```python
from build123d import *

# Parameters (mm, degrees)
SKETCH_1_R      = 5
SKETCH_1_R_2    = 3
EXTRUDE_1_DEPTH = 4
EXTRUDE_START   = 4
SKETCH_1_3_R    = 5
SKETCH_1_3_R_2  = 3
EXTRUDE_2_DEPTH = 2


with BuildPart() as part:
    # 草图1 → 凸台-拉伸1 (new body)
    # profile 1 of 2: a face of its own
    with BuildSketch(Plane(origin=(0, 0, 0), x_dir=(1, 0, 0), z_dir=(0, 1, 0))):
        with Locations(Location((0, 0, 0), (0, 0, 270))):
            Circle(SKETCH_1_R)
        with Locations(Location((0, 0, 0), (0, 0, 270))):
            Circle(SKETCH_1_R_2, mode=Mode.SUBTRACT)
    # profile 2 of 2: a face of its own
    with BuildSketch(Plane(origin=(0, 0, 0), x_dir=(1, 0, 0), z_dir=(0, 1, 0))):
        with Locations(Location((0, 0, 0), (0, 0, 270))):
            Circle(SKETCH_1_R_2)
        with BuildLine():
            ThreePointArc((-2, 1.5), (0, -2.5), (2, 1.5))
            Line((2, 1.5), (-2, 1.5))
        make_face(mode=Mode.SUBTRACT)
    extrude(amount=EXTRUDE_1_DEPTH)

    # 草图1<3> → 凸台-拉伸2 (add)
    with BuildSketch(Plane(origin=(0, 0, 0), x_dir=(1, 0, 0), z_dir=(0, 1, 0)).offset(EXTRUDE_START)):
        with Locations(Location((0, 0, 0), (0, 0, 270))):
            Circle(SKETCH_1_3_R)
        with Locations(Location((0, 0, 0), (0, 0, 270))):
            Circle(SKETCH_1_3_R_2, mode=Mode.SUBTRACT)
    extrude(amount=EXTRUDE_2_DEPTH)


solid = part.part
```
Source: CAD feature listing. Evaluate the final solid. Frame: model axes, mm. A direction names the side the tool comes from. Give positions to 0.01 mm unless a question says otherwise; leave off trailing zeros. Write each loop counter-clockwise with the first axis right and the second up, starting at its lowest first coordinate (ties: lowest second). Pieces come first, ordered by that corner, then holes. Notation, with made-up numbers: (29.5, 36.25) - (61.5, 36.25) arc R7 ccw to (61.5, 40.25) - close; hole circle Ø2 at (-15.75, 7.5). An arc over 180 degrees is marked (long way). One line per item, written item: value. Start each with the question number.
Q1. Draft query along X for faces 1 (the face through (-0.1, 2, 2.5)), 2 (the face through (-4.88, 2.96, -1.08)), 3 (the face through (0, 0, -2)). Return one class per face: +X half, -X half, draft (parallel to the pull), parting line (faces both ways), or undercut.
Q2. Section query C-C, the plane y = 2.25. Return the cut outline in (x, z).
Q3. Section query D-D, the plane z = -2. Return the cut outline in (x, y).
Q4. Section query B-B, the plane x = -1.25. Return the cut outline in (y, z), then the cut area to 3 significant figures.
Q5. Section query A-A, the plane z = 0. Return the cut outline in (x, y), then the cut area to 3 significant figures.
Q6. Material intervals for probe 1 along X at (y, z) = (2.9, 0); probe 2 along X at (y, z) = (4.4, 0); probe 3 along Z at (x, y) = (0.25, 0.5), sorted ascending. Write a range as from..to.
Q7. Set-up query: faces 4 (the face through (0.9, 4.99, 2.86)), 5 (the face through (0, 2, -1.5)), 6 (the face through (-3.3, 6, -0.1)). Return all of +Z, -Z, +X, -X, +Y, -Y with unobstructed straight access to the full face (end or side cutting, diameter ignored); none if empty.
Q8. First-contact query: pin 1 Ø3 at (x, y) = (-2.5, 0.5) entering from +Z; pin 2 Ø3 at (y, z) = (2.5, -0.5) entering from -X; pin 3 Ø1 at (y, z) = (4.5, -2) entering from -X. Flat tips, straight axial feed; report the tip coordinate or a pass-through.
Answer:
1. face 1: undercut
1. face 2: parting line
1. face 3: draft
2. outline: circle Ø10 at (0, 0); hole (-2, -1.5) - (2, -1.5) arc R2.5 ccw (long way) to start
3. outline: (-4.58, 0) - (4.58, 0) - (4.58, 6) - (2.24, 6) - (2.24, 4) - (-2.24, 4) - (-2.24, 6) - (-4.58, 6) - close
4. outline: (0, -4.84) - (6, -4.84) - (6, -2.73) - (4, -2.73) - (4, -1.5) - (0, -1.5) - close; (0, 2.17) - (4, 2.17) - (4, 2.73) - (6, 2.73) - (6, 4.84) - (0, 4.84) - close
4. area: 32.5 mm2
5. outline: (-5, 0) - (-2.5, 0) - (-2.5, 4) - (-3, 4) - (-3, 6) - (-5, 6) - close; (2.5, 0) - (5, 0) - (5, 6) - (3, 6) - (3, 4) - (2.5, 4) - close
5. area: 28.0 mm2
6. probe 1: x = -5..-2.5, 2.5..5
6. probe 2: x = -5..-3, 3..5
6. probe 3: z = -4.99..-1.5, 2.49..4.99
7. face 4: +Y
7. face 5: +Y, -Y
7. face 6: +Z, -Z, +X, -X, +Y
8. pin 1: stops at z = 4.9
8. pin 2: stops at x = -5
8. pin 3: stops at x = -4.77
